Input: part model. Units: mm. Frame: model coordinates. Face numbers are marked on the shaded views. A direction names the side the tool comes from. Round coordinates to 2 decimals unless told otherwise and drop trailing zeros. Write each loop counter-clockwise with the first axis right and the second up, starting at its lowest first coordinate (ties: lowest second). Pieces come first, ordered by that corner, then holes. Notation, with made-up numbers: M 22.5,64.25 L 60.5,64.25 A20 cw 60.5,91.25 Z; hole C 73.25,83 d4. An arc over 180 degrees is marked long. Answer as CSV lines item,"result". Start each with the question number.
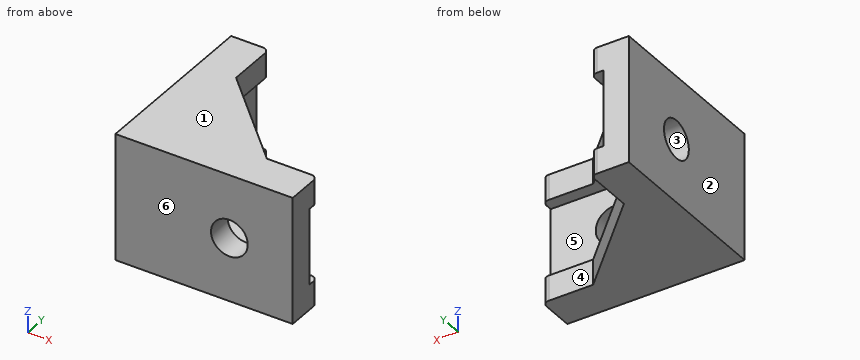
```python
from build123d import *

# Parameters (mm, degrees)
BOSS_EXTRUDE1_DEPTH = 20
SKETCH2_W           = 36.386493836
SKETCH2_H           = 30.590666468
CUT_EXTRUDE1_DEPTH  = 6
SKETCH4_R           = 3
CUT_EXTRUDE2_DEPTH  = 12
SKETCH5_R           = 2.9
CUT_EXTRUDE3_DEPTH  = 12
FILLET1_R           = 1


with BuildPart() as part:
    # Sketch1 → Boss-Extrude1 (new body)
    with BuildSketch(Plane.XY):
        Polygon((-25.115207597, 31.4260495), (-25.115207597, 3.4260495), (2.884792403, 3.4260495), (2.884792403, 9.4260495), (-5.115207597, 9.4260495), (-19.115207597, 23.4260495), (-19.115207597, 31.4260495), align=None)
    extrude(amount=BOSS_EXTRUDE1_DEPTH)

    # Sketch2 → Cut-Extrude1 (cut, symmetric)
    with BuildSketch(Plane.XY.offset(10)):
        with Locations((-2.921960679, 22.721382734)):
            Rectangle(SKETCH2_W, SKETCH2_H)
    extrude(amount=CUT_EXTRUDE1_DEPTH, both=True, mode=Mode.SUBTRACT)

    # Sketch4 → Cut-Extrude2 (cut)
    with BuildSketch(Plane(origin=(-21.115207597, 0, 0), x_dir=(0, 0, -1), z_dir=(1, 0, 0))):
        with Locations((-10, 19.9260495)):
            Circle(SKETCH4_R)
    extrude(amount=-CUT_EXTRUDE2_DEPTH, mode=Mode.SUBTRACT)

    # Sketch5 → Cut-Extrude3 (cut)
    with BuildSketch(Plane(origin=(0, 7.4260495, 0), x_dir=(1, 0, 0), z_dir=(0, 1, 0))):
        with Locations(Location((-7.115207597, -10, 0), (0, 0, 180))):
            Circle(SKETCH5_R)
    extrude(amount=-CUT_EXTRUDE3_DEPTH, mode=Mode.SUBTRACT)

    # Fillet1
    fillet1_edges = [part.edges().sort_by_distance(p)[0] for p in [
        (-19.115207597, 31.4260495, 18),
        (2.884792403, 9.4260495, 18),
        (-19.115207597, 31.4260495, 2),
        (2.884792403, 9.4260495, 2),
    ]]
    fillet(fillet1_edges, radius=FILLET1_R)


solid = part.part
```
Item 1: Line query: line 1 (Y direction, x = -24, z = 10); line 2 (X direction, y = 23.5, z = 11.5); line 3 (Z direction, x = -19, y = 23). Output: solid intervals per line, ascending. Write a range as [from, to].
Item 2: Pin query (flat end, axial travel): pin 1 Ø4.5 at (x, z) = (-7.12, 10) entering from -Y; pin 2 Ø1.2 at (x, z) = (-3, 1.5) entering from +Y; pin 3 Ø3.5 at (y, z) = (18, 9) entering from +X; pin 4 Ø5 at (y, z) = (19, 18) entering from +X. Return the tip coordinate at first contact, or that it passes through.
Item 3: Access query for the marked faces 4, 5 and 6. Directions: +Z, -Z, +X, -X, +Y, -Y. A direction counts if a zero-diameter tool reaches every point of the face in a straight line with its end or side. Return the directions, or none.
Item 4: Cut plane D-D, the plane z = 2.5. Return loops of the section in (x, y).
Item 5: Cut plane C-C, the plane y = 25.25. Return loops of the section in (x, z), plus the area to 3 significant figures.
Item 6: Cut plane B-B, the plane x = -7. Return loops of the section in (y, z).
Item 7: Draft query along Z for the marked faces 1, 2 and 3. Return one class per face: +Z half, -Z half, draft (parallel to the pull), parting line (faces both ways), or undercut.
Item 8: Cut plane A-A, the plane z = 10. Return loops of the section in (x, y).
Results list:
1,line 1,"[3.43, 16.93], [22.93, 31.43]"
1,line 2,"[-25.12, -21.12]"
1,line 3,"[0, 4], [16, 20]"
2,pin 1,"through"
2,pin 2,"y = 9.43"
2,pin 3,"x = -21.12"
2,pin 4,"x = -12.19"
3,face 4,"+Z, -Z, +X, +Y"
3,face 5,"+X, +Y"
3,face 6,"+Z, -Z, +X, -X, -Y"
4,outline,"M -25.12,3.43 L 2.88,3.43 L 2.88,8.43 A1 ccw 1.88,9.43 L -5.12,9.43 L -19.12,23.43 L -19.12,30.43 A1 ccw -20.12,31.43 L -25.12,31.43 Z"
5,outline,"M -25.12,0 L -19.12,0 L -19.12,4 L -21.12,4 L -21.12,16 L -19.12,16 L -19.12,20 L -25.12,20 Z"
5,area,"96.0 mm²"
6,outline,"M 3.43,0 L 11.31,0 L 11.31,4 L 7.43,4 L 7.43,7.1 L 3.43,7.1 Z; M 3.43,12.9 L 7.43,12.9 L 7.43,16 L 11.31,16 L 11.31,20 L 3.43,20 Z"
7,face 1,"+Z half"
7,face 2,"draft"
7,face 3,"undercut"
8,outline,"M -25.12,3.43 L -10.02,3.43 L -10.02,7.43 L -21.12,7.43 L -21.12,16.93 L -25.12,16.93 Z; M -25.12,22.93 L -21.12,22.93 L -21.12,31.43 L -25.12,31.43 Z; M -4.22,3.43 L 2.88,3.43 L 2.88,7.43 L -4.22,7.43 Z"
